Could you check a few things on this drawing? It's one solid part, dimensions in mm from its lowest x, y, z. A direction names the side the tool comes from. Round coordinates to 2 decimals unless told otherwise and drop trailing zeros. Write each loop counter-clockwise with the first axis right and the second up, starting at its lowest first coordinate (ties: lowest second). Pieces come first, ordered by that corner, then holes. Notation, with made-up numbers: (37.25, -38) -> (68.25, -38) arc R12 cw to (68.25, -27) -> close; hole circle Ø1 at (27.25, 0). An arc over 180 degrees is marked (long way). Return JSON: item names as keys, results as strings.
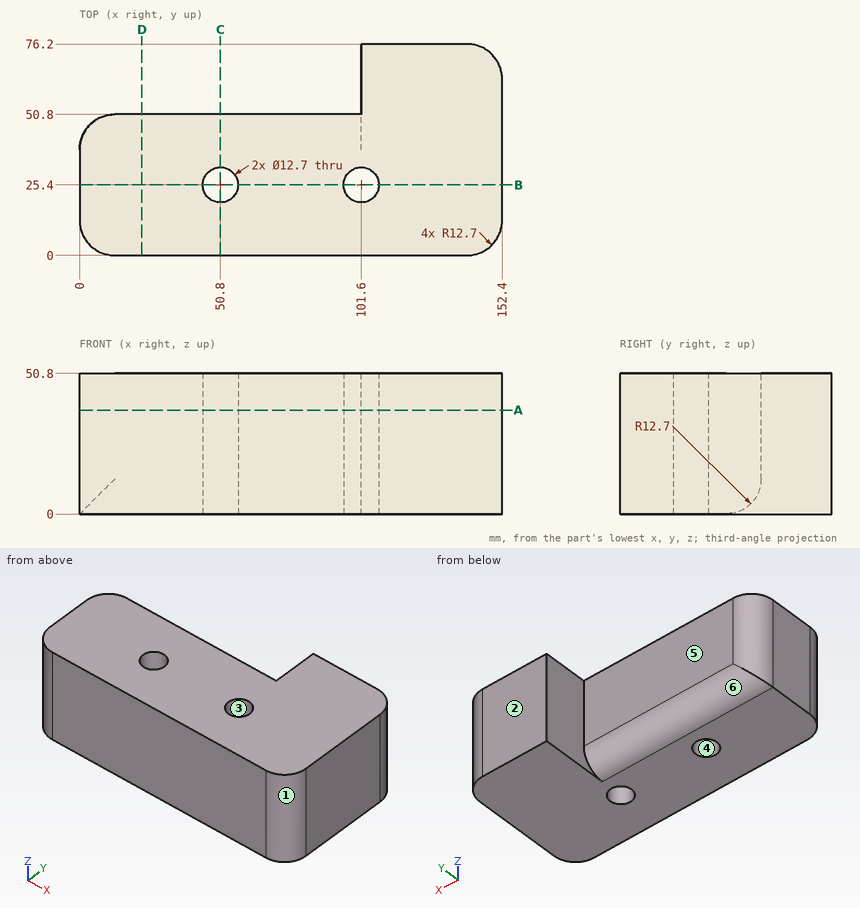
1) If I drill on probe 1 along X at (y, z) = (25, 27); probe 2 along X at (y, z) = (23, 32); probe 3 along Y at (x, z) = (50.8, 35.5), over which ranges is the centre line in solid material (lowest first)? Write a range as [from, to].
Return value:
{"probe 1": "[0, 44.46], [57.14, 95.26], [107.94, 152.4]", "probe 2": "[0, 44.92], [56.68, 95.72], [107.48, 152.4]", "probe 3": "[0, 19.05], [31.75, 50.8]"}
2) I want a section at D-D, the plane x = 22.5. Please give me the cut outline in (y, z).
Return value:
{"outline": "(0, 0) -> (38.1, 0) arc R12.7 ccw to (50.8, 12.7) -> (50.8, 50.8) -> (0, 50.8) -> close"}
3) I want a section at C-C, the plane x = 50.8. Please give me the cut outline in (y, z).
Return value:
{"outline": "(0, 0) -> (19.05, 0) -> (19.05, 50.8) -> (0, 50.8) -> close; (31.75, 0) -> (38.1, 0) arc R12.7 ccw to (50.8, 12.7) -> (50.8, 50.8) -> (31.75, 50.8) -> close"}
4) Will these pins go through, and if not, where does the flat tip stop? pin 1 Ø19 at (y, z) = (48, 22.5) entering from -X; pin 2 Ø4 at (y, z) = (44.5, 10.5) entering from -X; pin 3 Ø2 at (x, z) = (59.5, 39) entering from +Y; pin 4 Ø12 at (x, z) = (36, 17) entering from -Y.
Return value:
{"pin 1": "x = 0.01", "pin 2": "x = 0.79", "pin 3": "y = 50.8", "pin 4": "y = 0"}
5) For the marked faces 4, 5 and 6, which set-ups out of +Z, -Z, +X, -X, +Y, -Y let a thin tool reach every point of the face, with its end or its side?
Return value:
{"face 4": "+Z, -Z", "face 5": "+Z, -Z, -X, +Y", "face 6": "-Z, -X, +Y"}
6) Thinking about a two-plate mould opening in Y: for the marked faces 1, 2 and 3, which applies, pulls with the +Y half, pulls with the -Y half, needs draft (parallel to the pull), parting line crosses it, or undercut?
Return value:
{"face 1": "pulls with the -Y half", "face 2": "pulls with the +Y half", "face 3": "undercut"}
7) I want a section at B-B, the plane y = 25.4. Please give me the cut outline in (x, z), and give its area (3 significant figures).
Return value:
{"outline": "(0, 0) -> (44.45, 0) -> (44.45, 50.8) -> (0, 50.8) -> close; (57.15, 0) -> (95.25, 0) -> (95.25, 50.8) -> (57.15, 50.8) -> close; (107.95, 0) -> (152.4, 0) -> (152.4, 50.8) -> (107.95, 50.8) -> close", "area": "6,450 mm²"}
8) I want a section at A-A, the plane z = 37.5. Please give me the cut outline in (x, y), and give its area (3 significant figures).
Return value:
{"outline": "(0, 12.7) arc R12.7 ccw to (12.7, 0) -> (139.7, 0) arc R12.7 ccw to (152.4, 12.7) -> (152.4, 63.5) arc R12.7 ccw to (139.7, 76.2) -> (101.6, 76.2) -> (101.6, 50.8) -> (12.7, 50.8) arc R12.7 ccw to (0, 38.1) -> close; hole circle Ø12.7 at (50.8, 25.4); hole circle Ø12.7 at (101.6, 25.4)", "area": "8,640 mm²"}
